Verification items for the finished model (mm, model axes). A direction names the side the tool comes from. Give positions to 0.01 mm unless a question says otherwise; leave off trailing zeros. Loops run counter-clockwise (first coordinate to the right, second up) from the corner with the lowest first, then second, coordinate; pieces in that order, holes last. Notation, with made-up numbers: (10.5, 24) - (36.5, 24) arc R23 ccw to (36.5, 34) - close; hole circle Ø11 at (39, -14.75). An arc over 180 degrees is marked (long way). One line per item, written item: value. Start each with the question number.
1. Sectioned sample at D-D (y = 0). Record the cut outline in (x, z), plus the area to 3 significant figures.
2. Sectioned sample at C-C (y = -13). Record the cut outline in (x, z) (1 decimal), plus the area to 3 significant figures.
3. Access from +Z, -Z, +X, -X, +Y, -Y to the whole of each face (thin tool, end or side, straight path). Record for faces 1 (the flat face through (0, -22.225, 0)), 2 (the cylindrical face through (-3.78, -15.79, 2.9)), 3 (the cylindrical face through (-3.78, 19.7, 2.9)).
4. Sectioned sample at B-B (z = 0). Record the cut outline in (x, y) (1 decimal).
5. Gauge pin test, flat ends, axial feed: pin 1 (1 mm diameter, centred on y = 11, z = 3.5, fed in from -X); pin 2 (2 mm diameter, centred on x = -15.5, z = -5.5, fed in from -Y) (3 decimals); pin 3 (2 mm diameter, centred on y = 8.5, z = 9, fed in from -X). Record the tip position at first contact, or that the pin passes through.
6. Sectioned sample at A-A (x = 0). Record the cut outline in (y, z) (1 decimal), plus the area to 3 significant figures.
7. Scan lines: L1, parallel to Y at x = -10.5, z = 4.5 (3 decimals); L2, parallel to X at y = -3, z = -11.5; L3, parallel to Z at x = 2.5, y = -8. Record each from-to range of solid material in increasing order. Write a range as [from, to].
from build123d import *

# Parameters (mm, degrees)
SKETCH1_R           = 25.4
BOSS_EXTRUDE1_DEPTH = 9.525
SKETCH2_R           = 4.7625
BOSS_EXTRUDE2_DEPTH = 20.6375
SKETCH3_R           = 4.7625
CUT_EXTRUDE1_DEPTH  = 7.9375


with BuildPart() as part:
    # Sketch1 → Boss-Extrude1 (new body, symmetric)
    with BuildSketch(Plane(origin=(0, 0, 0), x_dir=(1, 0, 0), z_dir=(0, 1, 0))):
        Circle(SKETCH1_R)
    extrude(amount=BOSS_EXTRUDE1_DEPTH, both=True)

    # Sketch2 → Boss-Extrude2 (add)
    with BuildSketch(Plane(origin=(0, 9.525, 0), x_dir=(1, 0, 0), z_dir=(0, 1, 0))):
        Circle(SKETCH2_R)
    boss_extrude2 = extrude(amount=BOSS_EXTRUDE2_DEPTH)

    # Mirror1: Boss-Extrude2 across plane
    add(boss_extrude2.mirror(Plane.ZX))

    # Sketch3 → Cut-Extrude1 (cut)
    with BuildSketch(Plane(origin=(0, -30.1625, 0), x_dir=(-1, 0, 0), z_dir=(0, -1, 0))):
        Circle(SKETCH3_R)
    extrude(amount=-CUT_EXTRUDE1_DEPTH, mode=Mode.SUBTRACT)


solid = part.part
Results are:
1. outline: circle Ø50.8 at (0, 0)
1. area: 2,030 mm^2
2. outline: circle Ø9.5 at (0, 0)
2. area: 71.3 mm^2
3. face 1: +Z, -Z, +X, -X, -Y
3. face 2: -Y
3. face 3: +Y
4. outline: (-25.4, -9.5) - (-4.8, -9.5) - (-4.8, -22.2) - (4.8, -22.2) - (4.8, -9.5) - (25.4, -9.5) - (25.4, 9.5) - (4.8, 9.5) - (4.8, 30.2) - (-4.8, 30.2) - (-4.8, 9.5) - (-25.4, 9.5) - close
5. pin 1: stops at x = -3.7
5. pin 2: stops at y = -9.525
5. pin 3: stops at x = -24.11
6. outline: (-22.2, -4.8) - (-9.5, -4.8) - (-9.5, -25.4) - (9.5, -25.4) - (9.5, -4.8) - (30.2, -4.8) - (30.2, 4.8) - (9.5, 4.8) - (9.5, 25.4) - (-9.5, 25.4) - (-9.5, 4.8) - (-22.2, 4.8) - close
6. area: 1,290 mm^2
7. L1: y = [-9.525, 9.525]
7. L2: x = [-22.65, 22.65]
7. L3: z = [-25.28, 25.28]
